Can you work these out from the model? Positions are in its coordinate system, mm. A direction names the side the tool comes from. Round coordinates to 2 decimals unless told otherwise and drop trailing zeros. Write each loop counter-clockwise with the first axis right and the second up, starting at its lowest first coordinate (ties: lowest second). Pieces come first, ordered by that corner, then holes. Notation, with made-up numbers: (5.5, 64.25) -> (12.5, 64.25) arc R19 ccw to (12.5, 69.25) -> close; hole circle Ø9 at (30.5, 74.25). An arc over 180 degrees is marked (long way). Use CSV: the item, a comma, the result in double quotes.
```python
from build123d import *

# Parameters (mm, degrees)
F0_W      = 31.75
F0_H      = 31.75
F1_DEPTH  = 2.54
F2_R      = 28.829
F3_DEPTH  = 25.4
F4_DEPTH  = 2.54
F5_DEPTH  = 2.54
F6_DEPTH  = 2.54
F7_DEPTH  = 2.54
F8_R      = 31.369
F8_R_2    = 28.829
F9_DEPTH  = 19.05
F12_DEPTH = 2.54
F15_DEPTH = 2.54
F17_DEPTH = 3.175
F19_DEPTH = 3.175
F20_R     = 1.5875
F21_DEPTH = 25.4


# Not quite as in the source:
# - a pattern or mirror of a feature is missing from the dataset's text; its kind, count and spacing are read off the source's solid


with BuildPart() as f1:
    # F0 (on Top) → F1 (new body)
    with BuildSketch(Plane.XY):
        with Locations((-15.875, 15.875)):
            Rectangle(F0_W, F0_H)
        with Locations((15.875, -15.875)):
            Rectangle(F0_W, F0_H)
        with Locations((15.875, 15.875)):
            Rectangle(F0_W, F0_H)
        with Locations((-15.875, -15.875)):
            Rectangle(F0_W, F0_H)
    extrude(amount=F1_DEPTH)

    # F2 (on face) → F3 (cut)
    with BuildSketch(Plane.XY.offset(2.54)):
        Circle(F2_R)
    extrude(amount=-F3_DEPTH, mode=Mode.SUBTRACT)

    # F4 (add): a face of the model
    f4_faces = [f1.faces().sort_by_distance(p)[0] for p in [
        (0, -31.75, 1.27),
    ]]
    extrude(f4_faces, amount=F4_DEPTH)

    # F5 (add): a face of the model
    f5_faces = [f1.faces().sort_by_distance(p)[0] for p in [
        (0, 31.75, 1.27),
    ]]
    extrude(f5_faces, amount=F5_DEPTH)

    # F6 (add): a face of the model
    f6_faces = [f1.faces().sort_by_distance(p)[0] for p in [
        (31.75, 0, 1.27),
    ]]
    extrude(f6_faces, amount=F6_DEPTH)

    # F7 (add): a face of the model
    f7_faces = [f1.faces().sort_by_distance(p)[0] for p in [
        (-31.75, 0, 1.27),
    ]]
    extrude(f7_faces, amount=F7_DEPTH)

    # F8 (on face) → F9 (join)
    with BuildSketch(Plane.XY.offset(2.54)):
        Circle(F8_R)
        Circle(F8_R_2, mode=Mode.SUBTRACT)
    extrude(amount=F9_DEPTH)

    # F11 (on face) → F12 (join)
    with BuildSketch(Plane.XY.offset(2.54)):
        with BuildLine():
            Line((34.29, -34.29), (24.1616647691, -34.29))
            ThreePointArc((24.1616647691, -34.29), (36.604718933, -43.052889693), (34.29, -28.0109513551))
            Line((34.29, -28.0109513551), (34.29, -34.29))
        make_face()
    extrude(amount=-F12_DEPTH)

    # F13: F1 across plane


with BuildPart() as f1_1:
    add(f1.part)
    add(f1.part.mirror(Plane(origin=(0, 0, 1.27), x_dir=(0, -1, 0), z_dir=(-1, 0, 0))))

    # F14 (on face) → F15 (join)
    with BuildSketch(Plane.XY.offset(2.54)):
        with BuildLine():
            Line((34.29, 34.29), (34.29, 21.5044934303))
            ThreePointArc((34.29, 21.5044934303), (43.5698705735, 27.8972467151), (34.29, 34.29))
        make_face()
    extrude(amount=-F15_DEPTH)

    # F16: F1 across plane


with BuildPart() as f1_2:
    add(f1_1.part)
    add(f1_1.part.mirror(Plane(origin=(0, 0, 1.27), x_dir=(0, -1, 0), z_dir=(-1, 0, 0))))

    # F17 (add): a face of the model
    f17_faces = [f1_2.faces().sort_by_distance(p)[0] for p in [
        (0, -33.113583232, 0),
    ]]
    extrude(f17_faces, amount=F17_DEPTH)

    # F18 (on face) → F19 (cut)
    with BuildSketch(Plane(origin=(0, 0, -3.175), x_dir=(1, 0, 0), z_dir=(0, 0, -1))):
        with BuildLine():
            Line((0, 30.48), (-27.7283061296, 30.48))
            ThreePointArc((-27.7283061296, 30.48), (-35.4541518447, 42.4181121108), (-30.48, 29.0965121239))
            Line((-30.48, 29.0965121239), (-30.48, 3.2532289624))
            Line((-30.48, 3.2532289624), (-30.48, -27.1199196577))
            ThreePointArc((-30.48, -27.1199196577), (-42.2816797053, -26.6976345281), (-31.094558537, -30.48))
            Line((-31.094558537, -30.48), (0, -30.48))
            Line((0, -30.48), (0, 30.48))
        make_face()
    f19 = extrude(amount=-F19_DEPTH, mode=Mode.SUBTRACT)

    # F19_copies: F19 across plane
    add(f19.mirror(Plane(origin=(0, 0, 0), x_dir=(0, 0, 1), z_dir=(1, 0, 0))), mode=Mode.SUBTRACT)

    # F20 (on face) → F21 (cut)
    with BuildSketch(Plane(origin=(0, 0, 0), x_dir=(1, 0, 0), z_dir=(0, 0, -1))):
        with Locations((-32.3404680081, 36.1273235781)):
            Circle(F20_R)
        with Locations((32.3404680081, 36.1273235781)):
            Circle(F20_R)
        with Locations((36.8319889795, -27.8067924424)):
            Circle(F20_R)
        with Locations((-36.8319889795, -27.8067924424)):
            Circle(F20_R)
    extrude(amount=-F21_DEPTH, mode=Mode.SUBTRACT)


solid = f1_2.part
```
Q1. On a 3-axis mill with a long thin cutter (end or side, diameter ignored), from which of +Z, -Z, +X, -X, +Y, -Y can I reach the whole of each face in a straight line? I mean faces 1 (the face through (-30.48, -1, -2)), 2 (the face through (-6.8, -30.623, 11.932)), 3 (the face through (28, -9, 21.59)). Say none if no direction works.
Resolved:
face 1,"-Z"
face 2,"+Z"
face 3,"+Z, +X, -X, +Y, -Y"
Q2. Please list where these lines run through material, in increasing order: probe 1 along X at (y, z) = (12, -1.25); probe 2 along Y at (x, z) = (0, 10); probe 3 along Z at (x, y) = (4, -29).
Resolved:
probe 1,"x = -34.29 to -30.48, 30.48 to 34.29"
probe 2,"y = -31.37 to -28.83, 28.83 to 31.37"
probe 3,"z = 0 to 21.59"
Q3. Will these pins go through, and if not, where does the flat tip stop? P1, Ø5, axis at y = -8.5, z = 0.5, coming from the -X side; P2, Ø10.5, axis at x = 36.41, y = 27.77, coming from the -Z side; P3, Ø8, axis at x = -13, z = 13.5, coming from the -Y side.
Resolved:
P1,"stops at x = -34.29"
P2,"stops at z = 0"
P3,"stops at y = -30.05"
Q4. Suppose I cut it at C-C (z = 11.5). Write out the boundary of the cut face in (x, y).
Resolved:
outline,"circle Ø62.74 at (0, 0); hole circle Ø57.66 at (0, 0)"
Q5. Suppose I cut it at A-A (y = 0). Write out the boundary of the cut face in (x, z) (3 decimals).
Resolved:
outline,"(-34.29, -3.175) -> (-30.48, -3.175) -> (-30.48, 0) -> (-28.829, 0) -> (-28.829, 21.59) -> (-31.369, 21.59) -> (-31.369, 2.54) -> (-34.29, 2.54) -> close; (28.829, 0) -> (30.48, 0) -> (30.48, -3.175) -> (34.29, -3.175) -> (34.29, 2.54) -> (31.369, 2.54) -> (31.369, 21.59) -> (28.829, 21.59) -> close"
Q6. If we mould it in two halves opening along Y, with no side actions, what happens to faces 4 (the face through (34.29, -4, 0)), 5 (the face through (0, 34.29, 0)), 6 (the face through (0, 31, -3.175))? For each: released by +Y, released by -Y, zero draft, split by the parting line, or undercut.
Resolved:
face 4,"undercut"
face 5,"released by +Y"
face 6,"zero draft"
